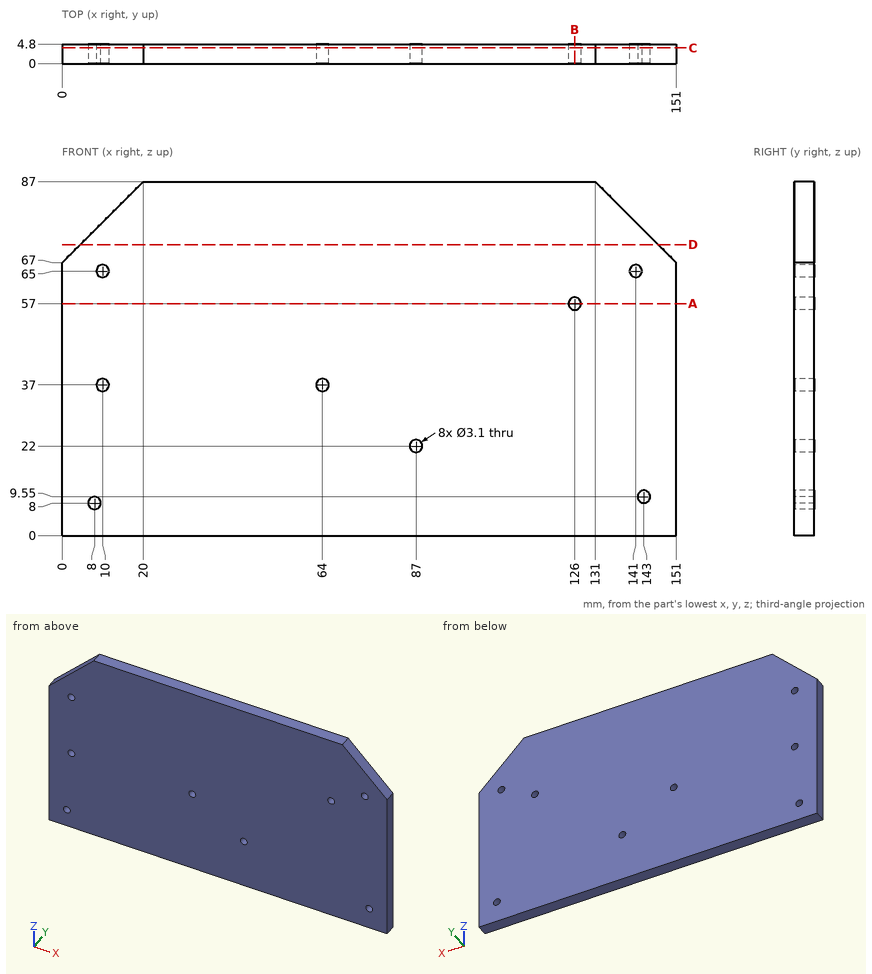
For this review, use the dimensioned drawing (mm, ordinates from the lowest corner) and the shaded views. Round coordinates to 2 decimals unless told otherwise and drop trailing zeros. Order: outer loops, then holes, each group sorted by start corner. A loop starts at its lowest first (then second) coordinate and runs counter-clockwise, first axis right, second up. Notation, with made-up numbers: M 79,81.5 L 121,81.5 A16 cw 121,92.5 Z; hole C 63.5,-32 d5. An arc over 180 degrees is marked long. Use a Markdown table: item, result.
1) Consider section D-D (z = 71.5). Write out the cut boundary in (x, y), then the cut area to 3 significant figures.
Report:
| item | result |
|---|---|
| outline | M 4.5,0 L 146.5,0 L 146.5,4.8 L 4.5,4.8 Z |
| area | 682 mm^2 |
2) Wall thickness on line 1 along X through (y, z) = (2.3, 65); line 2 along Z through (x, y) = (64, 2.1); line 3 along Z through (x, y) = (10, 2.45): over which ranges is each line inside the solid? List them lowest first. Write a range as [from, to].
Report:
| item | result |
|---|---|
| line 1 | [0, 8.45], [11.55, 139.45], [142.55, 151] |
| line 2 | [0, 35.45], [38.55, 87] |
| line 3 | [0, 35.45], [38.55, 63.45], [66.55, 77] |
3) Consider section C-C (y = 3.85). Give the number of separate pieces and of enclosed holes in the cut face, then the cut area to 3 significant figures.
Report:
| item | result |
|---|---|
| separate pieces | 1 |
| enclosed holes | 8 |
| area | 12,700 mm^2 |
4) Consider section B-B (x = 126). Write out the cut boundary in (y, z), then the cut area to 3 significant figures.
Report:
| item | result |
|---|---|
| outline | M 0,0 L 4.8,0 L 4.8,55.45 L 0,55.45 Z; M 0,58.55 L 4.8,58.55 L 4.8,87 L 0,87 Z |
| area | 403 mm^2 |
5) Insertion check: pin 1 (3.5 mm diameter, centred on x = 64, z = 37, fed in from +Y). The pin has a flat end and moves straight along its axis. Give the tip position at first contact, or say it passes through.
Report:
| item | result |
|---|---|
| pin 1 | y = 4.8 |
6) Consider section A-A (z = 57). Write out the cut boundary in (x, y).
Report:
| item | result |
|---|---|
| outline | M 0,0 L 124.45,0 L 124.45,4.8 L 0,4.8 Z; M 127.55,0 L 151,0 L 151,4.8 L 127.55,4.8 Z |
